Geometry: see drawing. Coordinates: mm, zero at the bounding-box minimum. A direction names the side the tool comes from. Round coordinates to 2 decimals unless told otherwise and drop trailing zeros. Order: outer loops, then holes, each group sorted by start corner. A loop starts at its lowest first (then second) coordinate and runs counter-clockwise, first axis right, second up.
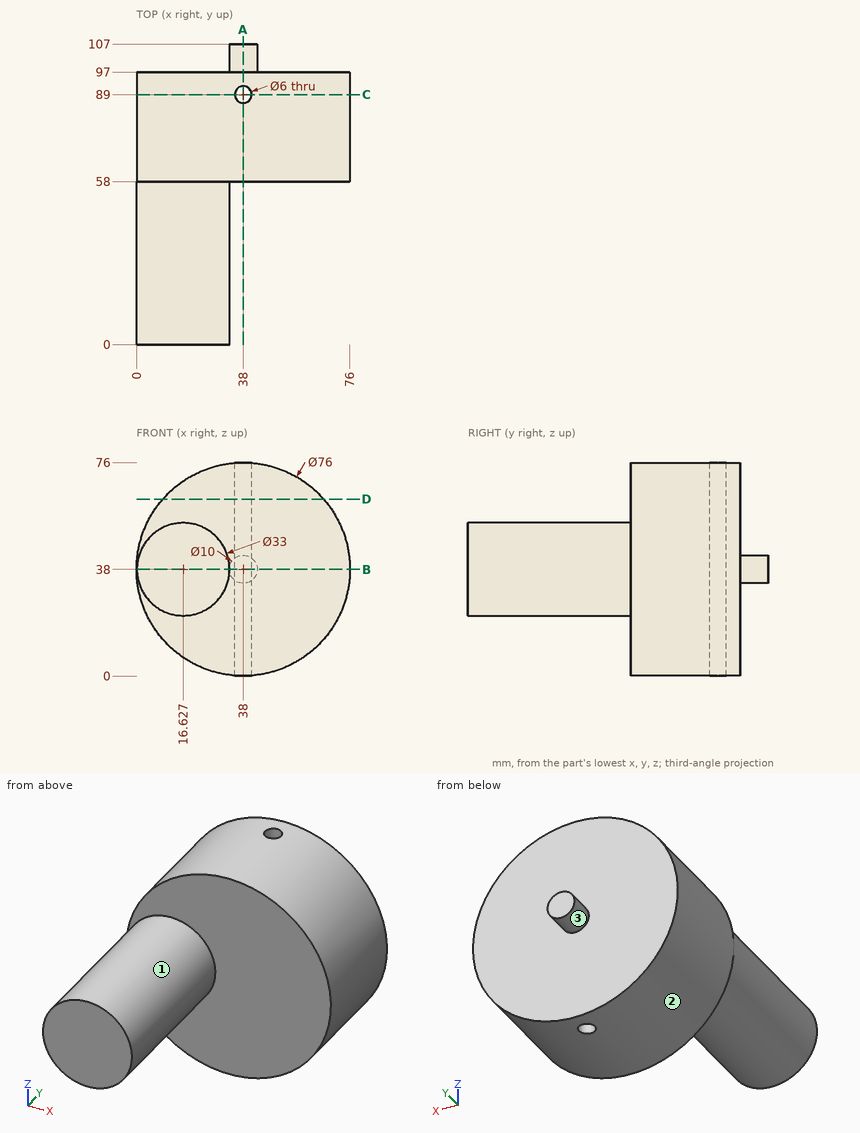
1. Section B-B on z = 38. Return loops of the section in (x, y).
2. Section C-C on y = 89. Return loops of the section in (x, z).
3. Access query for the marked faces 1, 2 and 3. Directions: +Z, -Z, +X, -X, +Y, -Y. A direction counts if a zero-diameter tool reaches every point of the face in a straight line with its end or side. Return the directions, or none.
4. First-contact query: pin 1 (4 mm diameter, centred on y = 59, z = 15, fed in from -X); pin 2 (2 mm diameter, centred on x = 12, z = 38, fed in from +Y); pin 3 (10 mm diameter, centred on x = 25.5, z = 63, fed in from -Y). Flat tips, straight axial feed; report the tip coordinate or a pass-through.
5. Section A-A on x = 38. Return loops of the section in (y, z), plus the area to 3 significant figures.
6. Section D-D on z = 63. Return loops of the section in (x, y), plus the area to 3 significant figures.
7. Line query: line 1 along Y through (x, z) = (38, 40); line 2 along Y through (x, z) = (49, 39.5); line 3 along X through (y, z) = (89, 48). Output: solid intervals per line, ascending.
Result:
1. outline: (0, 58) - (0.13, 58) - (0.13, 0) - (33.13, 0) - (33.13, 58) - (76, 58) - (76, 97) - (43, 97) - (43, 107) - (33, 107) - (33, 97) - (0, 97) - close; hole circle Ø6 at (38, 89)
2. outline: (35, 0.12) - (35, 75.88) arc R38 ccw to start; (41, 0.12) arc R38 ccw to (41, 75.88) - close
3. face 1: -Y
3. face 2: +Y, -Y
3. face 3: +Y
4. pin 1: stops at x = 6.33
4. pin 2: stops at y = 97
4. pin 3: stops at y = 58
5. outline: (58, 0) - (86, 0) - (86, 76) - (58, 76) - close; (92, 0) - (97, 0) - (97, 33) - (107, 33) - (107, 43) - (97, 43) - (97, 76) - (92, 76) - close
5. area: 2,610 mm2
6. outline: (9.38, 58) - (66.62, 58) - (66.62, 97) - (9.38, 97) - close; hole circle Ø6 at (38, 89)
6. area: 2,200 mm2
7. line 1: y = 58 to 86, 92 to 107
7. line 2: y = 58 to 97
7. line 3: x = 1.34 to 35, 41 to 74.66
